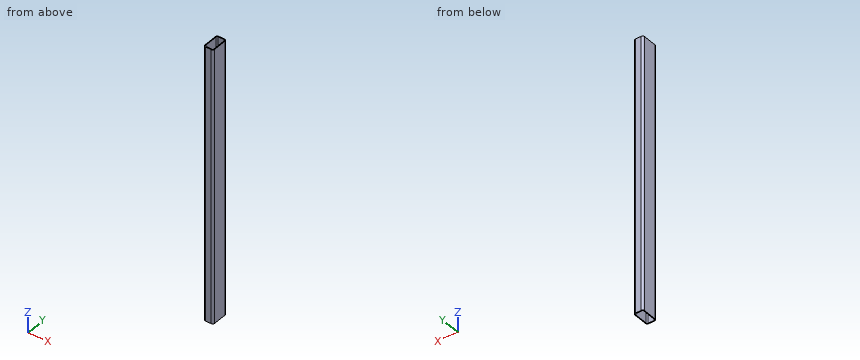
Autodesk Inventor part; units mm, degrees
ref_plane "Start Plane" through (0, 0, 60) normal (0, 0, 1) x (1, 0, 0)
ref_plane "End Plane" through (0, 0, 2940) normal (0, 0, 1) x (1, 0, 0)
ref_plane "Work Plane4" through (50, -1200, 60) normal (0, 0, -1) x (-1, 0, 0)
ref_plane "Start Plane" through (0, 0, 60) normal (0, 0, 1) x (1, 0, 0)
ref_plane "End Plane" through (0, 0, 2940) normal (0, 0, 1) x (1, 0, 0)
sketch "Sketch" plane through (0, 0, 0) normal (0, 0, 1) x (1, 0, 0)
  line L0 (-50, -70) -> (-50, 70)
  line L1 (-30, 90) -> (30, 90)
  line L2 (50, 70) -> (50, -70)
  line L3 (30, -90) -> (-30, -90)
  arc A0 (-50, -70) -> (-30, -90) centre (-30, -70) ccw
  arc A1 (50, 70) -> (30, 90) centre (30, 70) ccw
  arc A2 (-30, 90) -> (-50, 70) centre (-30, 70) ccw
  arc A3 (30, -90) -> (50, -70) centre (30, -70) ccw
  arc A4 (-30, 82) -> (-42, 70) centre (-30, 70) ccw
  line L4 (-30, 82) -> (30, 82)
  arc A5 (42, 70) -> (30, 82) centre (30, 70) ccw
  line L5 (42, 70) -> (42, -70)
  arc A6 (30, -82) -> (42, -70) centre (30, -70) ccw
  line L6 (30, -82) -> (-30, -82)
  arc A7 (-42, -70) -> (-30, -82) centre (-30, -70) ccw
  line L7 (-42, -70) -> (-42, 70)
  line L8 (0, 131.799) -> (0, -131.799) construction
  line L9 (-75.799, 0) -> (75.799, 0) construction
  dimension "d7" = 20
  dimension "d9" = 100
  dimension "d11" = 180
  dimension "d12" = 8
  dimension "d15" = 50
  dimension "d16" = 90
extrude "Body" add sketch "Sketch" along normal up to surface (2880 mm away) from surface at 60
sketch "Sketch3" plane through (0, 0, 0) normal (0, 0, 1) x (1, 0, 0)
  line L0 (0, 0) -> (10, 0)
ref_plane "Work Plane3" through (0, 0, 0) normal (0, -1, 0) x (1, 0, 0)
ref_plane "Work Plane4" through (50, -1200, 60) normal (0, 0, -1) x (-1, 0, 0)
split "Split1" plane through (50, -1200, 60) removes the side toward (0, 0, -1)
ref_plane "Work Plane5" through (-50, -1200, 2940) normal (0, 0, 1) x (1, 0, 0)
split "Split2" plane through (-50, -1200, 2940) removes the side toward (0, 0, 1)
sketch "Sketch4" plane through (0, 0, 0) normal (0, -1, 0) x (1, 0, 0)
  line L0 (-2, 60) -> (12, 60)
  line L1 (-2, 2940) -> (12, 2940)
  dimension "d18" = 2880
equation "\"d7\" = G_IR"
equation "\"d9\" = G_W"
equation "\"d11\" = G_H"
equation "\"d12\" = G_T"
equation "\"d15\" = 0.5 * d9"
equation "\"d16\" = 0.5 * d11"
equation "\"d3\" = G_L"
equation "\"G_W\" = 100"
equation "\"G_H\" = 180"
equation "\"G_T\" = 8"
equation "\"G_IR\" = 20"
equation "\"G_L\" = d18"
properties part number "ISO 10799-2 - 180x100x8 - 2880" material "Steel, Mild"
CAD build for the part. Positions are in the model's coordinates, mm. Coordinates: 2 decimals unless noted, no trailing zeros. Order: outer loops, then holes, each group sorted by start corner. A loop starts at its lowest first (then second) coordinate and runs counter-clockwise, first axis right, second up.
(1) Saw through at B-B, the plane z = 1078.5. Write the cut outline in (x, y), and give its area (3 significant figures).
Solution:
outline: (-50, -70) arc R20 ccw to (-30, -90) - (30, -90) arc R20 ccw to (50, -70) - (50, 70) arc R20 ccw to (30, 90) - (-30, 90) arc R20 ccw to (-50, 70) - close; hole (-42, -70) arc R12 ccw to (-30, -82) - (30, -82) arc R12 ccw to (42, -70) - (42, 70) arc R12 ccw to (30, 82) - (-30, 82) arc R12 ccw to (-42, 70) - close
area: 4,000 mm2
(2) Drill centre lines: L1, parallel to X at y = -13, z = 2438; L2, parallel to Y at x = 7, z = 2451.5; L3, parallel to Y at x = -36.5, z = 1800.5. Where is each one in solid material? Low to high.
Solution:
L1: x = -50 to -42, 42 to 50
L2: y = -90 to -82, 82 to 90
L3: y = -88.91 to -80.09, 80.09 to 88.91
(3) Pin check, flat tips, straight feed: pin 1 Ø1.5 at (x, z) = (-38.5, 1616.5) entering from -Y; pin 2 Ø2 at (x, z) = (37.5, 2209.5) entering from -Y; pin 3 Ø3 at (x, z) = (-34, 2012.5) entering from +Y. Stop position of each tip, or through.
Solution:
pin 1: stops at y = -88.44
pin 2: stops at y = -88.91
pin 3: stops at y = 89.84
(4) Saw through at C-C, the plane x = 0. Write the cut outline in (y, z).
Solution:
outline: (-90, 60) - (-82, 60) - (-82, 2940) - (-90, 2940) - close; (82, 60) - (90, 60) - (90, 2940) - (82, 2940) - close
(5) Saw through at A-A, the plane y = -22. Write the cut outline in (x, z), and give its area (3 significant figures).
Solution:
outline: (-50, 60) - (-42, 60) - (-42, 2940) - (-50, 2940) - close; (42, 60) - (50, 60) - (50, 2940) - (42, 2940) - close
area: 46,100 mm2
